Design review of the part built by this model. Coordinates are the model's own, in mm. Give positions to 0.01 mm unless a question says otherwise; leave off trailing zeros. Write each loop counter-clockwise with the first axis right and the second up, starting at its lowest first coordinate (ties: lowest second). Pieces come first, ordered by that corner, then holes. Notation, with made-up numbers: M -35.5,15 L 15.5,15 A38 cw 15.5,54 Z; hole C 74.25,64.25 d5. An arc over 180 degrees is marked long. Answer in a Markdown table with one row per item.
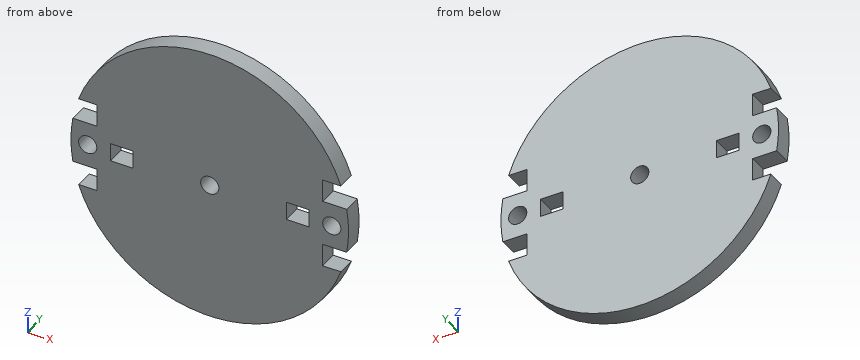
```python
from build123d import *

# Parameters (mm, degrees)
CROQUIS1_R              = 30.5
SALIENTE_EXTRUIR1_DEPTH = 4
CROQUIS2_R              = 2
CORTAR_EXTRUIR1_DEPTH   = 4
CORTAR_EXTRUIR3_START   = -4
CORTAR_EXTRUIR3_DEPTH   = 4
CROQUIS6_W              = 5
CROQUIS6_H              = 4
CORTAR_EXTRUIR4_DEPTH   = 4
CROQUIS7_R              = 2
CORTAR_EXTRUIR5_DEPTH   = 4


with BuildPart() as part:
    # Croquis1 → Saliente-Extruir1 (new body)
    with BuildSketch(Plane(origin=(0, 0, 0), x_dir=(1, 0, 0), z_dir=(0, 1, 0))):
        with Locations(Location((0, 0, 0), (0, 0, 270))):
            Circle(CROQUIS1_R)
    extrude(amount=SALIENTE_EXTRUIR1_DEPTH)

    # Croquis2 → Cortar-Extruir1 (cut)
    with BuildSketch(Plane(origin=(0, 4, 0), x_dir=(1, 0, 0), z_dir=(0, 1, 0))):
        with Locations(Location((0, 0, 0), (0, 0, 270))):
            Circle(CROQUIS2_R)
    extrude(amount=-CORTAR_EXTRUIR1_DEPTH, mode=Mode.SUBTRACT)

    # Croquis5 → Cortar-Extruir3 (cut)
    with BuildSketch(Plane(origin=(0, 4, 0), x_dir=(1, 0, 0), z_dir=(0, 1, 0)).offset(CORTAR_EXTRUIR3_START)):
        with BuildLine():
            Line((28.814059068, 5), (30.087372767, 5))
            ThreePointArc((30.087372767, 5), (29.556634924, 7.526973624), (28.814059068, 10))
            Line((28.814059068, 10), (24.814059068, 10))
            Line((24.814059068, 10), (24.814059068, 5))
            Line((24.814059068, 5), (28.814059068, 5))
        make_face()
        with BuildLine():
            Line((30.087372767, -5), (28.814059068, -5))
            Line((28.814059068, -5), (24.814059068, -5))
            Line((24.814059068, -5), (24.814059068, -10))
            Line((24.814059068, -10), (28.814059068, -10))
            ThreePointArc((28.814059068, -10), (29.556634924, -7.526973624), (30.087372767, -5))
        make_face()
        with BuildLine():
            Line((-24.814059068, 5), (-24.814059068, 10))
            Line((-24.814059068, 10), (-28.814059068, 10))
            ThreePointArc((-28.814059068, 10), (-29.556634924, 7.526973624), (-30.087372767, 5))
            Line((-30.087372767, 5), (-28.814059068, 5))
            Line((-28.814059068, 5), (-24.814059068, 5))
        make_face()
        with BuildLine():
            Line((-28.814059068, -10), (-24.814059068, -10))
            Line((-24.814059068, -10), (-24.814059068, -5))
            Line((-24.814059068, -5), (-28.814059068, -5))
            Line((-28.814059068, -5), (-30.087372767, -5))
            ThreePointArc((-30.087372767, -5), (-29.556634924, -7.526973624), (-28.814059068, -10))
        make_face()
    extrude(amount=CORTAR_EXTRUIR3_DEPTH, mode=Mode.SUBTRACT)

    # Croquis6 → Cortar-Extruir4 (cut)
    with BuildSketch(Plane(origin=(0, 4, 0), x_dir=(1, 0, 0), z_dir=(0, 1, 0))):
        with Locations((-19.314059068, 0)):
            Rectangle(CROQUIS6_W, CROQUIS6_H)
        with Locations((19.314059068, 0)):
            Rectangle(CROQUIS6_W, CROQUIS6_H)
    extrude(amount=-CORTAR_EXTRUIR4_DEPTH, mode=Mode.SUBTRACT)

    # Croquis7 → Cortar-Extruir5 (cut)
    with BuildSketch(Plane(origin=(0, 4, 0), x_dir=(1, 0, 0), z_dir=(0, 1, 0))):
        with Locations(Location((-26.814059068, 0, 0), (0, 0, 270))):
            Circle(CROQUIS7_R)
        with Locations(Location((26.814059068, 0, 0), (0, 0, 90))):
            Circle(CROQUIS7_R)
    extrude(amount=-CORTAR_EXTRUIR5_DEPTH, mode=Mode.SUBTRACT)


solid = part.part
```
1) To check wall thickness, follow probe 1 along X at (y, z) = (3.25, 0); probe 2 along Z at (x, y) = (27, 0.9); probe 3 along X at (y, z) = (2.35, 6.5). State the ranges of each line that lie inside material, in increasing order. Write a range as [from, to].
Geometry says:
| item | result |
|---|---|
| probe 1 | [-30.5, -28.81], [-24.81, -21.81], [-16.81, -2], [2, 16.81], [21.81, 24.81], [28.81, 30.5] |
| probe 2 | [-14.19, -10], [-5, -1.99], [1.99, 5], [10, 14.19] |
| probe 3 | [-24.81, 24.81] |
2) Add section C-C (y = 2.5). Write out the cut boundary in (x, z), and give its area (3 significant figures).
Geometry says:
| item | result |
|---|---|
| outline | M -30.09,-5 L -24.81,-5 L -24.81,-10 L -28.81,-10 A30.5 ccw 28.81,-10 L 24.81,-10 L 24.81,-5 L 30.09,-5 A30.5 ccw 30.09,5 L 24.81,5 L 24.81,10 L 28.81,10 A30.5 ccw -28.81,10 L -24.81,10 L -24.81,5 L -30.09,5 A30.5 ccw Z; hole C -26.81,0 d4; hole M -21.81,-2 L -16.81,-2 L -16.81,2 L -21.81,2 Z; hole C 0,0 d4; hole M 16.81,-2 L 21.81,-2 L 21.81,2 L 16.81,2 Z; hole C 26.81,0 d4 |
| area | 2,750 mm^2 |
3) Insertion check: P1, Ø6, axis at x = -1, z = 2.5, coming from the -Y side; P2, Ø2, axis at x = 29, y = 1.5, coming from the +Z side; P3, Ø1.2, axis at x = 26, y = 1, coming from the +Z side; P4, Ø2, axis at x = -4, y = 2.5, coming from the -Z side. Each pin has a flat end and moves straight along its axis. Give the tip position at first contact, or say it passes through.
Geometry says:
| item | result |
|---|---|
| P1 | y = 0 |
| P2 | z = 12.09 |
| P3 | z = 16.88 |
| P4 | z = -30.35 |
4) Add section A-A (z = 0). Write out the cut boundary in (x, y).
Geometry says:
| item | result |
|---|---|
| outline | M -30.5,0 L -28.81,0 L -28.81,4 L -30.5,4 Z; M -24.81,0 L -21.81,0 L -21.81,4 L -24.81,4 Z; M -16.81,0 L -2,0 L -2,4 L -16.81,4 Z; M 2,0 L 16.81,0 L 16.81,4 L 2,4 Z; M 21.81,0 L 24.81,0 L 24.81,4 L 21.81,4 Z; M 28.81,0 L 30.5,0 L 30.5,4 L 28.81,4 Z |
5) Add section D-D (z = -7). Write out the cut boundary in (x, y), and give its area (3 significant figures).
Geometry says:
| item | result |
|---|---|
| outline | M -24.81,0 L 24.81,0 L 24.81,4 L -24.81,4 Z |
| area | 199 mm^2 |
6) Add section B-B (x = 0). Write out the cut boundary in (y, z).
Geometry says:
| item | result |
|---|---|
| outline | M 0,-30.5 L 4,-30.5 L 4,-2 L 0,-2 Z; M 0,2 L 4,2 L 4,30.5 L 0,30.5 Z |
